Part model, mm, in its own coordinate system. Face numbers are marked on the shaded views. Give positions to 0.01 mm unless a question says otherwise; leave off trailing zeros. Write each loop counter-clockwise with the first axis right and the second up, starting at its lowest first coordinate (ties: lowest second). Pieces come first, ordered by that corner, then holes.
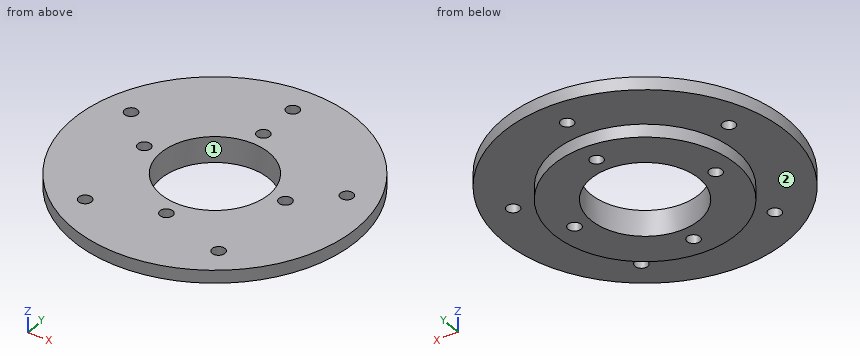
from build123d import *

# Parameters (mm, degrees)
F0_R     = 34.925
F0_R_2   = 1.5875
F0_R_3   = 13.335
F1_DEPTH = 6.35
F2_R     = 34.925
F2_R_2   = 22.5
F3_DEPTH = 3.175


with BuildPart() as f1:
    # F0 (on Top) → F1 (new body)
    with BuildSketch(Plane.XY):
        Circle(F0_R)
        with Locations((-16.42272, -22.603935)):
            Circle(F0_R_2, mode=Mode.SUBTRACT)
        with Locations((16.42272, -22.603935)):
            Circle(F0_R_2, mode=Mode.SUBTRACT)
        with Locations((0, -17.375)):
            Circle(F0_R_2, mode=Mode.SUBTRACT)
        with Locations((-26.572519, 8.633935)):
            Circle(F0_R_2, mode=Mode.SUBTRACT)
        with Locations((-17.375, 0)):
            Circle(F0_R_2, mode=Mode.SUBTRACT)
        Circle(F0_R_3, mode=Mode.SUBTRACT)
        with Locations((17.375, 0)):
            Circle(F0_R_2, mode=Mode.SUBTRACT)
        with Locations((0, 17.375)):
            Circle(F0_R_2, mode=Mode.SUBTRACT)
        with Locations((26.572519, 8.633935)):
            Circle(F0_R_2, mode=Mode.SUBTRACT)
        with Locations((0, 27.94)):
            Circle(F0_R_2, mode=Mode.SUBTRACT)
    extrude(amount=F1_DEPTH)

    # F2 (on face) → F3 (cut)
    with BuildSketch(Plane(origin=(0, 0, 0), x_dir=(1, 0, 0), z_dir=(0, 0, -1))):
        Circle(F2_R)
        Circle(F2_R_2, mode=Mode.SUBTRACT)
    extrude(amount=-F3_DEPTH, mode=Mode.SUBTRACT)


solid = f1.part
1) Flat gauge pins, fed straight in: P1, Ø1, axis at x = -26, y = -9.5, coming from the -Z side (3 decimals); P2, Ø3, axis at y = 22.5, z = 2, coming from the +X side; P3, Ø3, axis at y = 26, z = 5, coming from the -X side. Where does each tip first touch, or does it go through?
Check result:
P1: stops at z = 3.175
P2: stops at x = 27.47
P3: stops at x = -24.89
2) Drill centre lines: L1, parallel to Y at x = 0, z = 5.25 (1 decimal); L2, parallel to Y at x = -1, z = 2; L3, parallel to X at y = 0.5, z = 2.5. Where is each one in solid material? Low to high.
Check result:
L1: y = -34.9 to -19, -15.8 to -13.3, 13.3 to 15.8, 19 to 26.4, 29.5 to 34.9
L2: y = -22.48 to -18.61, -16.14 to -13.3, 13.3 to 16.14, 18.61 to 22.48
L3: x = -22.49 to -18.88, -15.87 to -13.33, 13.33 to 15.87, 18.88 to 22.49
3) Saw through at C-C (y = -7.5). Write the cut outline in (x, z) (3 decimals), and give its area (3 significant figures).
Check result:
outline: (-34.11, 3.175) - (-21.213, 3.175) - (-21.213, 0) - (-11.026, 0) - (-11.026, 6.35) - (-34.11, 6.35) - close; (11.026, 0) - (21.213, 0) - (21.213, 3.175) - (34.11, 3.175) - (34.11, 6.35) - (11.026, 6.35) - close
area: 211 mm2
4) Mould opens along Y. For the marked faces 1 and 2 say: +Y half, -Y half, draft (parallel to the pull), parting line (faces both ways), or undercut.
Check result:
face 1: undercut
face 2: draft
5) Saw through at A-A (y = 0). State how many separate pieces and enclosed holes the cut face has, and give its area (3 significant figures).
Check result:
separate pieces: 4
enclosed holes: 0
area: 155 mm2
